Input: part model. Units: mm. Frame: model coordinates. A direction names the side the tool comes from. Round coordinates to 2 decimals unless told otherwise and drop trailing zeros. Loops run counter-clockwise (first coordinate to the right, second up) from the corner with the lowest first, then second, coordinate; pieces in that order, holes last.
1) Draft query along X for faces 5 (the face through (6, 40, 624)), 6 (the face through (231.5, -32, 968)), 7 (the face through (128, 95, 415.5)), 8 (the face through (49, 6, 626)). Return one class per face: pulls with the +X half, pulls with the -X half, needs draft (parallel to the pull), parting line crosses it, or undercut.
2) Section A-A, the plane x = 50. Return loops of the section in (y, z).
3) Section C-C, the plane z = 789.5. Return loops of the section in (x, y), and give its area (3 significant figures).
4) Section B-B, the plane x = 160. State how many separate pieces and enclosed holes the cut face has, and give its area (3 significant figures).
5) Access query for faces 1 (the face through (139, 56, 751)), 2 (the face through (252, -45, 1003)), 3 (the face through (128, 81.5, 429)), 4 (the face through (246.5, -27, 968)). Directions: +Z, -Z, +X, -X, +Y, -Y. A direction counts if a zero-diameter tool reaches every point of the face in a straight line with its end or side. Return the directions, or none.
6) First-contact query: pin 1 (24 mm diameter, centred on x = 246.5, y = -28.5, fed in from -Z); pin 2 (10 mm diameter, centred on x = 231.5, y = -22.5, fed in from +Z); pin 3 (8 mm diameter, centred on x = 70.5, z = 986.5, fed in from +Y). Flat tips, straight axial feed; report the tip coordinate or a pass-through.
7) Ray query, line 1 along Y through (x, z) = (160, 894.25); line 2 along Z through (x, y) = (171.5, 46.5); line 3 along Y through (x, z) = (57.5, 237). Return the intervals inside material, ascending.
8) Section D-D, the plane z = 143. Return loops of the section in (x, y), and give its area (3 significant figures).
from build123d import *
from OCP.BRepFilletAPI import BRepFilletAPI_MakeChamfer

# Parameters (mm, degrees)
SCHIZZO1_W                      = 88
SCHIZZO1_H                      = 68
ESTRUSIONE_SOTTILE1_DEPTH       = 1200
ESTRUSIONE1_DEPTH               = 1207.813987324
SCHIZZO4_R                      = 15
ESTRUSIONE3_DEPTH               = 12
SCHIZZO5_W                      = 15
SCHIZZO5_H                      = 70
ESTRUSIONE4_DEPTH               = 30
ESTRUSIONE5_DEPTH               = 10
SCHIZZO8_R                      = 12
ESTRUSIONE6_DEPTH               = 1244.48542412
SMUSSO1_SIZE                    = 60
SMUSSO1_SIZE2                   = 34.641016151
SMUSSO2_SIZE                    = 10
SMUSSO2_SIZE2                   = 13.08013562
RACCORDO1_R                     = 8
SCHIZZO9_R                      = 6
ESTRUSIONE7_DEPTH               = 1222.90670675
SCHIZZO10_R                     = 10
ESTRUSIONE8_DEPTH               = 10
ESTRUSIONE_SOTTILE2_DEPTH       = 150
ESTRUSIONE_SOTTILE2_DEPTH_BACK  = 90
SCHIZZO11_W                     = 27
SCHIZZO11_H                     = 27
SCHIZZO12_W                     = 8
SCHIZZO12_H                     = 40
ESTRUSIONE_ESTRUSIONE1_DEPTH    = 80
SCHIZZO13_R                     = 12
TAGLIO_ESTRUSIONE1_DEPTH        = 894.050950394
RACCORDO2_R                     = 10
RIPETIZIONE_A_L1_COUNT          = 2
RIPETIZIONE_A_L1_PITCH          = 149
RACCORDO2_OF_RIPETIZIONE_A_L1_R = 10
SCHIZZO14_R                     = 7
ESTRUSIONE_ESTRUSIONE2_DEPTH    = 20
TAGLIO_ESTRUSIONE2_START        = 670
SCHIZZO15_R                     = 4
TAGLIO_ESTRUSIONE2_DEPTH        = 250


with BuildPart() as part:
    # Schizzo1 → Estrusione-Sottile1 (new body)
    with BuildSketch(Plane.XY):
        with BuildLine():
            Line((5, 0), (95, 0))
            ThreePointArc((95, 0), (98.535533906, 1.464466094), (100, 5))
            Line((100, 5), (100, 75))
            ThreePointArc((100, 75), (98.535533906, 78.535533906), (95, 80))
            Line((95, 80), (5, 80))
            ThreePointArc((5, 80), (1.464466094, 78.535533906), (0, 75))
            Line((0, 75), (0, 5))
            ThreePointArc((0, 5), (1.464466094, 1.464466094), (5, 0))
        make_face()
        with Locations((50, 40)):
            Rectangle(SCHIZZO1_W, SCHIZZO1_H, mode=Mode.SUBTRACT)
    extrude(amount=ESTRUSIONE_SOTTILE1_DEPTH)

    # Schizzo2 → Estrusione1 (cut, through all)
    with BuildSketch(Plane(origin=(100, 0, 0), x_dir=(0, 0, -1), z_dir=(1, 0, 0))):
        Polygon((-1200, 80), (-1050, 0), (-1200, 0), align=None)
        Polygon((-64, 80), (-214, 0), (0, 0), (0, 80), align=None)
    extrude(amount=-ESTRUSIONE1_DEPTH, mode=Mode.SUBTRACT)

    # Schizzo4 → Estrusione3 (add)
    with BuildSketch(Plane.XZ):
        Polygon((5, 1050), (100, 1050), (316, 1003), (316, 890), (95, 890), (5, 890), align=None)
        with Locations(Location((286.5, 973, 0), (0, 0, 270))):
            Circle(SCHIZZO4_R, mode=Mode.SUBTRACT)
    extrude(amount=ESTRUSIONE3_DEPTH)

    # Schizzo5 → Estrusione4 (add)
    with BuildSketch(Plane.XZ.offset(12)):
        with Locations((239, 968)):
            Rectangle(SCHIZZO5_W, SCHIZZO5_H)
    extrude(amount=ESTRUSIONE4_DEPTH)

    # Schizzo7 → Estrusione5 (add)
    with BuildSketch(Plane.XZ.offset(42)):
        Polygon((231.5, 1003), (316, 1003), (316, 943), (261.5, 943), (261.5, 933), (231.5, 933), align=None)
    extrude(amount=ESTRUSIONE5_DEPTH)

    # Schizzo8 → Estrusione6 (cut, through all)
    with BuildSketch(Plane(origin=(0, 0, 0), x_dir=(1, 0, 0), z_dir=(0, 1, 0))):
        with Locations(Location((286.5, -973, 0), (0, 0, 270))):
            Circle(SCHIZZO8_R)
    extrude(amount=-ESTRUSIONE6_DEPTH, mode=Mode.SUBTRACT)

    # Smusso1
    smusso1_edges = [part.edges().sort_by_distance(p)[0] for p in [
        (316, -6, 890),
    ]]
    smusso1_side = [part.faces().sort_by_distance(p)[0] for p in [
        (160.5, -6, 890),
    ]]
    chamfer(smusso1_edges, length=SMUSSO1_SIZE, length2=SMUSSO1_SIZE2, reference=smusso1_side[0])

    # Smusso2: one chamfer whose edges measure the first distance from different faces: ONE call of the kernel's chamfer builder (chamfer() names one face for all edges)
    smusso2_edges_1 = [part.edges().sort_by_distance(p)[0] for p in [
        (316, -6, 1003),
    ]]
    smusso2_side_1 = [part.faces().sort_by_distance(p)[0] for p in [
        (316, -6, 963.820508076),
    ]]
    smusso2_edges_2 = [part.edges().sort_by_distance(p)[0] for p in [
        (316, -47, 1003),
        (316, -47, 943),
    ]]
    smusso2 = BRepFilletAPI_MakeChamfer(part.part.solid().wrapped)
    for e in smusso2_edges_1:
        smusso2.Add(SMUSSO2_SIZE, SMUSSO2_SIZE2, e.wrapped, smusso2_side_1[0].wrapped)  # the first distance lies on this face
    for e in smusso2_edges_2:
        smusso2.Add(SMUSSO2_SIZE, e.wrapped)
    add(Compound.cast(smusso2.Shape()), mode=Mode.REPLACE)

    # Raccordo1
    raccordo1_edges = [part.edges().sort_by_distance(p)[0] for p in [
        (261.5, -47, 933),
    ]]
    fillet(raccordo1_edges, radius=RACCORDO1_R)

    # Schizzo9 → Estrusione7 (cut, through all)
    with BuildSketch(Plane(origin=(100, 0, 0), x_dir=(0, 0, -1), z_dir=(1, 0, 0))):
        with Locations((-254, 55)):
            Circle(SCHIZZO9_R)
    extrude(amount=-ESTRUSIONE7_DEPTH, mode=Mode.SUBTRACT)

    # Schizzo10 → Estrusione8 (cut)
    with BuildSketch(Plane(origin=(100, 0, 0), x_dir=(0, 0, -1), z_dir=(1, 0, 0))):
        with Locations((-254, 55)):
            Circle(SCHIZZO10_R)
    extrude(amount=-ESTRUSIONE8_DEPTH, mode=Mode.SUBTRACT)

    # Schizzo11 → Estrusione-Sottile2 (add, two sides: drawn at the far end of the back side and taken through both)
    with BuildSketch(Plane(origin=(100, 0, 0), x_dir=(0, 0, -1), z_dir=(1, 0, 0)).offset(-ESTRUSIONE_SOTTILE2_DEPTH_BACK)):
        with BuildLine():
            Line((-442.5, 110), (-415.5, 110))
            ThreePointArc((-415.5, 110), (-414.439339828, 109.560660172), (-414, 108.5))
            Line((-414, 108.5), (-414, 81.5))
            ThreePointArc((-414, 81.5), (-414.439339828, 80.439339828), (-415.5, 80))
            Line((-415.5, 80), (-442.5, 80))
            ThreePointArc((-442.5, 80), (-443.560660172, 80.439339828), (-444, 81.5))
            Line((-444, 81.5), (-444, 108.5))
            ThreePointArc((-444, 108.5), (-443.560660172, 109.560660172), (-442.5, 110))
        make_face()
        with Locations((-429, 95)):
            Rectangle(SCHIZZO11_W, SCHIZZO11_H, mode=Mode.SUBTRACT)
    extrude(amount=ESTRUSIONE_SOTTILE2_DEPTH + ESTRUSIONE_SOTTILE2_DEPTH_BACK)

    # Schizzo12 → Estrusione-Estrusione1 (add)
    with BuildSketch(Plane(origin=(100, 0, 0), x_dir=(0, 0, -1), z_dir=(1, 0, 0))):
        with Locations((-896, 56)):
            Rectangle(SCHIZZO12_W, SCHIZZO12_H)
    estrusione_estrusione1 = extrude(amount=ESTRUSIONE_ESTRUSIONE1_DEPTH)

    # Schizzo13 → Taglio-Estrusione1 (cut, through all)
    with BuildSketch(Plane(origin=(0, 0, 892), x_dir=(-1, 0, 0), z_dir=(0, 0, -1))):
        with Locations((-160, 56)):
            Circle(SCHIZZO13_R)
    taglio_estrusione1 = extrude(amount=-TAGLIO_ESTRUSIONE1_DEPTH, mode=Mode.SUBTRACT)

    # Raccordo2
    raccordo2_edges = [part.edges().sort_by_distance(p)[0] for p in [
        (180, 36, 896),
        (180, 76, 896),
    ]]
    fillet(raccordo2_edges, radius=RACCORDO2_R)

    # Ripetizione a L1: Estrusione-Estrusione1, Taglio-Estrusione1 ×2
    with Locations(*[(0, 0, -i * RIPETIZIONE_A_L1_PITCH) for i in range(1, RIPETIZIONE_A_L1_COUNT)]):
        add(estrusione_estrusione1)
        add(taglio_estrusione1, mode=Mode.SUBTRACT)

    # Raccordo2 of Ripetizione a L1
    raccordo2_of_ripetizione_a_l1_edges = [part.edges().sort_by_distance(p)[0] for p in [
        (180, 36, 747),
        (180, 76, 747),
    ]]
    fillet(raccordo2_of_ripetizione_a_l1_edges, radius=RACCORDO2_OF_RIPETIZIONE_A_L1_R)

    # Schizzo14 → Estrusione-Estrusione2 (add)
    with BuildSketch(Plane(origin=(0, 80, 0), x_dir=(1, 0, 0), z_dir=(0, 1, 0))):
        with Locations((88, -821)):
            Circle(SCHIZZO14_R)
    extrude(amount=ESTRUSIONE_ESTRUSIONE2_DEPTH)

    # Schizzo15 → Taglio-Estrusione2 (cut)
    with BuildSketch(Plane.XY.offset(TAGLIO_ESTRUSIONE2_START)):
        with Locations(Location((88, 93, 0), (0, 0, 180))):
            Circle(SCHIZZO15_R)
    extrude(amount=TAGLIO_ESTRUSIONE2_DEPTH, mode=Mode.SUBTRACT)


solid = part.part
Final values:
1. face 5: undercut
1. face 6: pulls with the -X half
1. face 7: needs draft
1. face 8: undercut
2. outline: (-12, 890) - (0, 890) - (0, 214) - (6, 202.75) - (6, 1061.25) - (0, 1050) - (-12, 1050) - close; (74, 75.25) - (80, 64) - (80, 415.5) arc R1.5 ccw to (81.5, 414) - (108.5, 414) arc R1.5 ccw to (110, 415.5) - (110, 442.5) arc R1.5 ccw to (108.5, 444) - (81.5, 444) arc R1.5 ccw to (80, 442.5) - (80, 1200) - (74, 1188.75) - close; hole (81.5, 415.5) - (108.5, 415.5) - (108.5, 442.5) - (81.5, 442.5) - close
3. outline: (0, 5) arc R5 ccw to (5, 0) - (95, 0) arc R5 ccw to (100, 5) - (100, 75) arc R5 ccw to (95, 80) - (5, 80) arc R5 ccw to (0, 75) - close; hole (6, 6) - (94, 6) - (94, 74) - (6, 74) - close
3. area: 1,990 mm2
4. separate pieces: 6
4. enclosed holes: 1
4. area: 2,190 mm2
5. face 1: +X, +Y, -Y
5. face 2: +Z, +X, -X, -Y
5. face 3: +X, -X
5. face 4: +Z, -Z, +X
6. pin 1: stops at z = 933
6. pin 2: stops at z = 1003
6. pin 3: stops at y = 80
7. line 1: y = -12 to 0, 36 to 44, 68 to 76
7. line 2: z = 743 to 751, 892 to 900
7. line 3: y = 0 to 6, 74 to 80
8. outline: (0, 37.87) - (6, 37.87) - (6, 74) - (94, 74) - (94, 37.87) - (100, 37.87) - (100, 75) arc R5 ccw to (95, 80) - (5, 80) arc R5 ccw to (0, 75) - close
8. area: 1,020 mm2
